Geometry check sheet. Reference: the model listing, model coordinates, mm. A direction names the side the tool comes from. Round coordinates to 2 decimals unless told otherwise and drop trailing zeros. Write each loop counter-clockwise with the first axis right and the second up, starting at its lowest first coordinate (ties: lowest second). Pieces come first, ordered by that corner, then holes. Notation, with made-up numbers: M -14.75,54.25 L 27.25,54.25 A22 cw 27.25,82.25 Z; hole C -9,89 d5. An arc over 180 degrees is marked long. One line per item, written item: value. Start each with the question number.
1. Section check B-B (y = 5.5). Record the boundary of the cut face in (x, z).
2. Release check for a two-part mould opening along Y. For faces 3 (the cylindrical face through (1.479, 5.268, -0.163)), 4 (the flat face through (-6, -3, 0)), 5 (the flat face through (3, 4, 0)), 6 (the cylindrical face through (1.52, 7.14, -9.1)) record: pulls with the +Y half, pulls with the -Y half, needs draft (parallel to the pull), parting line crosses it, or undercut.
3. Access from +Z, -Z, +X, -X, +Y, -Y to the whole of each face (thin tool, end or side, straight path). Record for faces 1 (the flat face through (-2, -1, -10)), 2 (the flat face through (0, 4, 0)).
4. Section check C-C (x = -9.25). Record the boundary of the cut face in (y, z).
5. Section check A-A (z = 0). Record the boundary of the cut face in (x, y).
6. Scan lines: probe 1 along X at (y, z) = (6.75, -5); probe 2 along Y at (x, z) = (-4.25, 0); probe 3 along Y at (x, z) = (0.75, 0). Record each from-to range of solid material in increasing order. Write a range as [from, to].
7. Depth check by flat-ended pin: P1, Ø6, axis at x = -7, z = -0.5, coming from the +Y side; P2, Ø2.5, axis at x = -9, z = 6, coming from the -Y side; P3, Ø6, axis at y = 4.5, z = -4, coming from the -X side. Enter the tip coordinate at first touch or a pass-through.
8. Section check D-D (y = -1). Record the boundary of the cut face in (x, z), and give its area (3 significant figures).
from build123d import *

# Parameters (mm, degrees)
BASE_FLANGE1_DEPTH = 10
FILLET1_R          = 3
SKETCH6_R          = 1.5
CUT_EXTRUDE1_DEPTH = 18.549928775
SKETCH7_R          = 0.75
CUT_EXTRUDE2_DEPTH = 18.549928775


# Sheet-metal steps are written as plain solids
with BuildPart() as part:
    # Sketch1 → Base-Flange1 (new, symmetric)
    with BuildSketch(Plane.XY):
        with BuildLine():
            Line((-12, 0), (-0.75, 0))
            ThreePointArc((-0.75, 0), (-0.219669914, 0.219669914), (0, 0.75))
            Line((0, 0.75), (0, 8))
            Line((0, 8), (3, 8))
            Line((3, 8), (3, 0.75))
            ThreePointArc((3, 0.75), (1.901650429, -1.901650429), (-0.75, -3))
            Line((-0.75, -3), (-12, -3))
            Line((-12, -3), (-12, 0))
        make_face()
    extrude(amount=BASE_FLANGE1_DEPTH, both=True)

    # Fillet1
    fillet1_edges = [part.edges().sort_by_distance(p)[0] for p in [
        (-12, -1.5, 10),
        (-12, -1.5, -10),
        (1.5, 8, 10),
        (1.5, 8, -10),
    ]]
    fillet(fillet1_edges, radius=FILLET1_R)

    # Sketch6 → Cut-Extrude1 (cut, through all)
    with BuildSketch(Plane(origin=(0, 0, 0), x_dir=(1, 0, 0), z_dir=(0, 1, 0))):
        with Locations(Location((-9, 6, 0), (0, 0, 270))):
            Circle(SKETCH6_R)
        with Locations(Location((-9, -6, 0), (0, 0, 90))):
            Circle(SKETCH6_R)
    extrude(amount=-CUT_EXTRUDE1_DEPTH, mode=Mode.SUBTRACT)

    # Sketch7 → Cut-Extrude2 (cut, through all)
    with BuildSketch(Plane.ZY):
        with Locations((0, 6)):
            Circle(SKETCH7_R)
    extrude(amount=-CUT_EXTRUDE2_DEPTH, mode=Mode.SUBTRACT)


solid = part.part
Result sheet:
1. outline: M 0,-9.96 L 3,-9.96 L 3,-0.56 L 0,-0.56 Z; M 0,0.56 L 3,0.56 L 3,9.96 L 0,9.96 Z
2. face 3: undercut
2. face 4: pulls with the -Y half
2. face 5: needs draft
2. face 6: pulls with the +Y half
3. face 1: -Z, +X, -X, +Y, -Y
3. face 2: +Z, -Z, -X, +Y
4. outline: M -3,-9.99 L 0,-9.99 L 0,-7.48 L -3,-7.48 Z; M -3,-4.52 L 0,-4.52 L 0,4.52 L -3,4.52 Z; M -3,7.48 L 0,7.48 L 0,9.99 L -3,9.99 Z
5. outline: M -12,-3 L -0.75,-3 A3.75 ccw 3,0.75 L 3,5.25 L 0,5.25 L 0,0.75 A0.75 cw -0.75,0 L -12,0 Z; M 0,6.75 L 3,6.75 L 3,8 L 0,8 Z
6. probe 1: x = [0, 3]
6. probe 2: y = [-3, 0]
6. probe 3: y = [-2.69, 5.25], [6.75, 8]
7. P1: stops at y = 0
7. P2: passes through
7. P3: stops at x = 0
8. outline: M -12,-7 A3 ccw -9,-10 L 2.57,-10 L 2.57,10 L -9,10 A3 ccw -12,7 Z; hole C -9,-6 d3; hole C -9,6 d3
8. area: 273 mm2
